Build history of the part. All positions in model axes, mm. A direction names the side the tool comes from. Give positions to 0.01 mm unless a question says otherwise; leave off trailing zeros. Write each loop counter-clockwise with the first axis right and the second up, starting at its lowest first coordinate (ties: lowest second). Pieces come first, ordered by that corner, then holes.
Autodesk Inventor part; units mm, degrees
ref_plane "YZ Plane" through (0, 0, 0) normal (1, 0, 0) x (0, 1, 0)
ref_plane "XZ Plane" through (0, 0, 0) normal (0, 1, 0) x (-1, 0, 0)
ref_plane "XY Plane" through (0, 0, 0) normal (0, 0, 1) x (1, 0, 0)
sketch "Sketch1" plane through (0, 0, 0) normal (0, 0, 1) x (1, 0, 0)
  circle A0 centre (0, 0) radius 16.75
  line L0 (0, 0) -> (-17.65, 0) construction
  line L1 (-15.7399, -5.7288) -> (0, 0) construction
  line L2 (-14.2048, -8.8761) -> (0, 0) construction
  line L3 (-46, -6) -> (-46, -24)
  line L4 (-36.3668, 2) -> (-36.3668, -10)
  line L5 (-36.3668, -10) -> (-27.3668, -10)
  line L6 (-36.3668, -20) -> (-29.8668, -20)
  line L7 (-36.3668, -20) -> (-36.3668, -32)
  line L8 (-17.5898, -16) -> (-17.5898, -16)
  arc A1 (-27.3668, -10) -> (-22, 0) centre (-34, 0) ccw
  line L9 (34.6332, -10.9067) -> (34.6332, 21.7526) construction
  line L10 (115.2665, -6) -> (115.2665, -24)
  arc A2 (105.6332, -32) -> (115.2665, -24) centre (107.128, -24) ccw
  line L11 (105.6332, 2) -> (105.6332, -10)
  line L12 (105.6332, -10) -> (96.6332, -10)
  line L13 (105.6332, -20) -> (99.1332, -20)
  line L14 (105.6332, -20) -> (105.6332, -32)
  line L15 (96.6332, -10) -> (96.6332, 14)
  line L16 (0, 22) -> (88.6332, 22)
  line L17 (99.1332, -20) -> (94.6332, -20)
  line L18 (86.6332, -12) -> (86.6332, 4)
  line L19 (78.6332, 12) -> (29.7321, 12)
  arc A3 (96.6332, 14) -> (88.6332, 22) centre (88.6332, 14) ccw
  arc A4 (86.6332, 4) -> (78.6332, 12) centre (78.6332, 4) ccw
  arc A5 (86.6332, -12) -> (94.6332, -20) centre (94.6332, -12) ccw
  arc A6 (-6.3721, -21.057) -> (21.8036, 2.9333) centre (0, 0) ccw
  arc A7 (0, 22) -> (-22, 0) centre (0, 0) ccw
  arc A8 (29.7321, 12) -> (21.8036, 2.9333) centre (29.7321, 4) ccw
  line L20 (-19.8668, -27) -> (-29.8668, -27)
  line L21 (-29.8668, -27) -> (-29.8668, -20)
  line L22 (-46, -15) -> (-35.8797, -15) construction
  arc A9 (-6.3721, -21.057) -> (-18.1004, -25.9381) centre (-9.2685, -30.6283) ccw
  arc A10 (-19.8668, -27) -> (-18.1004, -25.9381) centre (-19.8668, -25) ccw
  arc A11 (-46, -24) -> (-36.3668, -32) centre (-37.8615, -24) ccw
  arc A12 (-36.3668, 2) -> (-46, -6) centre (-37.8615, -6) ccw
  arc A13 (115.2665, -6) -> (105.6332, 2) centre (107.128, -6) ccw
  point P0 (18.4391, 12)
  point P1 (-18.5871, -27)
  dimension "d12" = 16.75
  dimension "d19" = 160
  dimension "d30" = 9
  dimension "d40" = 46
  dimension "d43" = 8
  dimension "d44" = 22
  dimension "d45" = 8
  dimension "d46" = 10
  dimension "d47" = 10
  dimension "d48" = 142
  dimension "d59" = 6.5
  dimension "d61" = 10
  dimension "d63" = 12
  dimension "d65" = 10
  dimension "d66" = 2
  dimension "d67" = 10
  dimension "d68" = 10
  dimension "d69" = 7
  dimension "d70" = 5
  dimension "d71" = 12
  dimension "d72" = 18
extrude "Extrusion1" add sketch "Sketch1" along normal blind 5.85
properties part number "waterbottle_holder"
(1) Saw through at B-B, the plane y = -4.5. List the corners of the cut face in (x, z).
(2) Probe line 1 (Y direction, x = 0, z = 3.45); line 2 (X direction, y = -12, z = 1.6); line 3 (X direction, y = -4, z = 3). List the from-to ranges inside material, lowest first.
(3) Saw through at A-A, the plane y = -15. List the corners of the cut face in (x, z).
(4) Mould opens along Y. For faces 4 (the face through (100, -20, 3)), 5 (the face through (-3.63, 16.35, 2.88)), 6 (the face through (16, 7, 0)), 7 (the face through (-15.73, 15.38, 2.88)) say: +Y half, -Y half, draft (parallel to the pull), parting line (faces both ways), or undercut.
(5) 3-axis set-ups, long thin cutter, end or side, ignore diameter. For faces 1 (the face through (96.633, 2, 3)), 2 (the face through (-46, -15, 3)), 3 (the face through (86.633, -4, 3)): which of +Z, -Z, +X, -X, +Y, -Y reach the whole face in a straight line?
(6) Drop flat-ended pins along their axis: pin 1 (3 mm diameter, centred on y = 4, z = 2, fed in from +X); pin 2 (1.8 mm diameter, centred on y = -24.5, z = 4, fed in from -X); pin 3 (1.8 mm diameter, centred on x = 98.5, z = 2, fed in from -Y); pin 4 (1.8 mm diameter, centred on y = -2, z = 4, fed in from -X). Give the stop position or say it passes through.
(7) Saw through at D-D, the plane x = 69.5. List the corners of the cut face in (y, z).
Computed values:
1. outline: (-45.86, 0) - (-36.37, 0) - (-36.37, 5.85) - (-45.86, 5.85) - close; (-22.88, 0) - (-16.13, 0) - (-16.13, 5.85) - (-22.88, 5.85) - close; (16.13, 0) - (21.53, 0) - (21.53, 5.85) - (16.13, 5.85) - close; (86.63, 0) - (96.63, 0) - (96.63, 5.85) - (86.63, 5.85) - close; (105.63, 0) - (115.13, 0) - (115.13, 5.85) - (105.63, 5.85) - close
2. line 1: y = -22 to -16.75, 16.75 to 22
2. line 2: x = -46 to -11.69, 11.69 to 18.44, 86.63 to 115.27
2. line 3: x = -45.75 to -36.37, -22.69 to -16.27, 16.27 to 21.63, 86.63 to 96.63, 105.63 to 115.02
3. outline: (-46, 0) - (-7.45, 0) - (-7.45, 5.85) - (-46, 5.85) - close; (7.45, 0) - (16.09, 0) - (16.09, 5.85) - (7.45, 5.85) - close; (87.22, 0) - (115.27, 0) - (115.27, 5.85) - (87.22, 5.85) - close
4. face 4: -Y half
4. face 5: undercut
4. face 6: draft
4. face 7: +Y half
5. face 1: +Z, -Z, +Y
5. face 2: +Z, -Z, -X, +Y, -Y
5. face 3: +Z, -Z, -Y
6. pin 1: stops at x = 96.63
6. pin 2: stops at x = -46
6. pin 3: stops at y = -20
6. pin 4: stops at x = -45.39
7. outline: (12, 0) - (22, 0) - (22, 5.85) - (12, 5.85) - close
